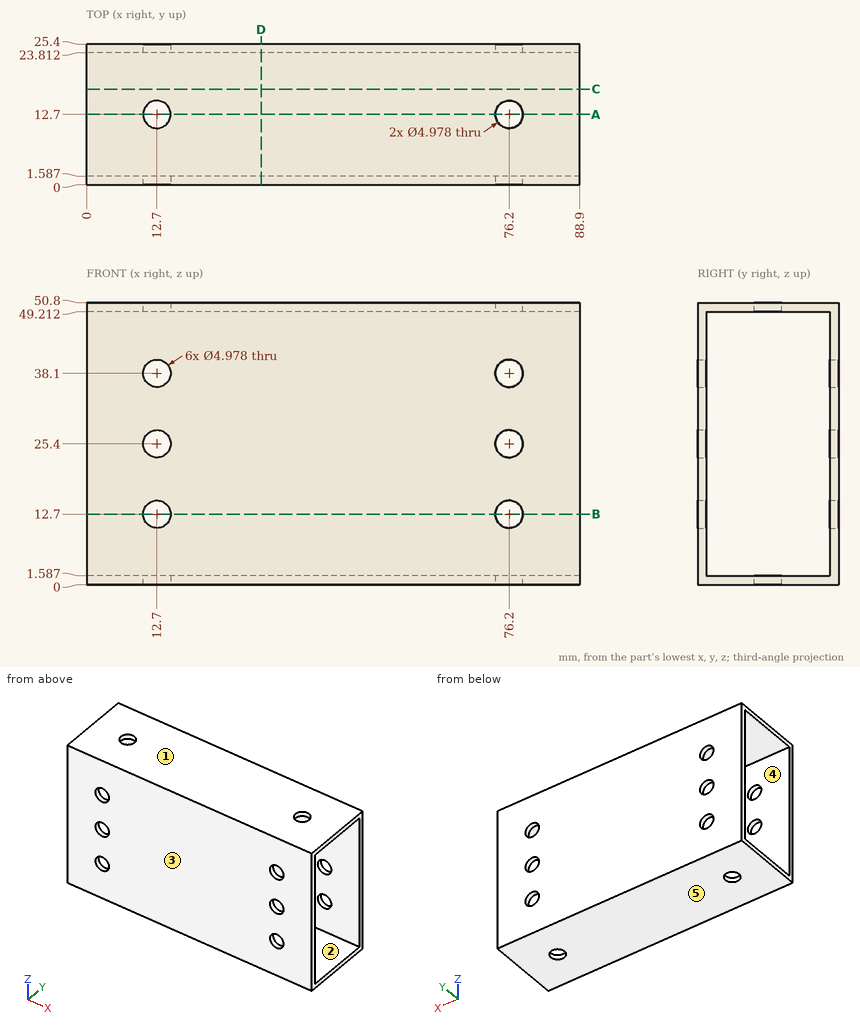
For this review, use the dimensioned drawing (mm, ordinates from the lowest corner) and the shaded views. A direction names the side the tool comes from. Give positions to 0.01 mm unless a question says otherwise; leave off trailing zeros. Order: outer loops, then holes, each group sorted by start corner. A loop starts at its lowest first (then second) coordinate and runs counter-clockwise, first axis right, second up.
1) Take a section at C-C (y = 17.25). Give the boundary of the cut face in (x, z).
2) Take a section at A-A (y = 12.7). Give the boundary of the cut face in (x, z).
3) Wall thickness on line 1 (Z direction, x = 12.7, y = 0.85); line 2 (X direction, y = 24.7, z = 12.7); line 3 (Z direction, x = 67, y = 14.25): over which ranges is each line inside the solid? List them lowest first.
4) For the marked faces 4 and 5, list the 3-axis set-ups (+Z, -Z, +X, -X, +Y, -Y) from which the entire face can be reached by the end or side of a thin tool; tool diameter is ignored.
5) Take a section at D-D (x = 31.5). Give the boundary of the cut face in (y, z).
6) Take a section at B-B (z = 12.7). Give the boundary of the cut face in (x, y).
7) Insertion check: pin 1 (4 mm diameter, centred on x = 12.7, y = 12.7, fed in from -Z); pin 2 (3 mm diameter, centred on x = 64, y = 13.5, fed in from -Z). Each pin has a flat end and moves straight along its axis. Give the tip position at first contact, or say it passes through.
8) The part is to be moulded in two halves that separate along Y. For the marked faces 1, 2 and 3, say which applies: released by +Y, released by -Y, zero draft, split by the parting line, or undercut.
Derived:
1. outline: (0, 0) - (88.9, 0) - (88.9, 1.59) - (0, 1.59) - close; (0, 49.21) - (88.9, 49.21) - (88.9, 50.8) - (0, 50.8) - close
2. outline: (0, 0) - (10.21, 0) - (10.21, 1.59) - (0, 1.59) - close; (0, 49.21) - (10.21, 49.21) - (10.21, 50.8) - (0, 50.8) - close; (15.19, 0) - (73.71, 0) - (73.71, 1.59) - (15.19, 1.59) - close; (15.19, 49.21) - (73.71, 49.21) - (73.71, 50.8) - (15.19, 50.8) - close; (78.69, 0) - (88.9, 0) - (88.9, 1.59) - (78.69, 1.59) - close; (78.69, 49.21) - (88.9, 49.21) - (88.9, 50.8) - (78.69, 50.8) - close
3. line 1: z = 0 to 10.21, 15.19 to 22.91, 27.89 to 35.61, 40.59 to 50.8
3. line 2: x = 0 to 10.21, 15.19 to 73.71, 78.69 to 88.9
3. line 3: z = 0 to 1.59, 49.21 to 50.8
4. face 4: +X, -X
4. face 5: -Z, +X, -X, +Y, -Y
5. outline: (0, 0) - (25.4, 0) - (25.4, 50.8) - (0, 50.8) - close; hole (1.59, 1.59) - (23.81, 1.59) - (23.81, 49.21) - (1.59, 49.21) - close
6. outline: (0, 0) - (10.21, 0) - (10.21, 1.59) - (0, 1.59) - close; (0, 23.81) - (10.21, 23.81) - (10.21, 25.4) - (0, 25.4) - close; (15.19, 0) - (73.71, 0) - (73.71, 1.59) - (15.19, 1.59) - close; (15.19, 23.81) - (73.71, 23.81) - (73.71, 25.4) - (15.19, 25.4) - close; (78.69, 0) - (88.9, 0) - (88.9, 1.59) - (78.69, 1.59) - close; (78.69, 23.81) - (88.9, 23.81) - (88.9, 25.4) - (78.69, 25.4) - close
7. pin 1: passes through
7. pin 2: stops at z = 0
8. face 1: zero draft
8. face 2: undercut
8. face 3: released by -Y
